from build123d import *

# Parameters (mm, degrees)
SKETCH1_W           = 155
SKETCH1_H           = 55
SKETCH1_R           = 3.25
BOSS_EXTRUDE1_DEPTH = 10
CUT_EXTRUDE1_DEPTH  = 7
SKETCH3_R           = 2.5
CUT_EXTRUDE2_DEPTH  = 10
FILLET1_R           = 3


with BuildPart() as part:
    # Sketch1 → Boss-Extrude1 (new body)
    with BuildSketch(Plane.XY):
        with Locations((2.15707133, 4.04038984)):
            Rectangle(SKETCH1_W, SKETCH1_H)
        with Locations((-45.34292867, 4.04038984)):
            Circle(SKETCH1_R, mode=Mode.SUBTRACT)
        with Locations((-8.34292867, 4.04038984)):
            Circle(SKETCH1_R, mode=Mode.SUBTRACT)
        with Locations((55.65707133, 6.54038984)):
            Circle(SKETCH1_R, mode=Mode.SUBTRACT)
    extrude(amount=BOSS_EXTRUDE1_DEPTH)

    # Sketch2 → Cut-Extrude1 (cut)
    with BuildSketch(Plane.XY.offset(10)):
        with BuildLine():
            Line((-75.34292867, 31.54038984), (-63.34292867, 31.54038984))
            Line((-63.34292867, 31.54038984), (-63.34292867, 24.04038984))
            ThreePointArc((-63.34292867, 24.04038984), (-64.660948155, 20.858409325), (-67.84292867, 19.54038984))
            Line((-67.84292867, 19.54038984), (-75.34292867, 19.54038984))
            Line((-75.34292867, 19.54038984), (-75.34292867, 31.54038984))
        make_face()
        with BuildLine():
            Line((-75.34292867, -23.45961016), (-63.34292867, -23.45961016))
            Line((-63.34292867, -23.45961016), (-63.34292867, -15.95961016))
            ThreePointArc((-63.34292867, -15.95961016), (-64.660948155, -12.777629645), (-67.84292867, -11.45961016))
            Line((-67.84292867, -11.45961016), (-75.34292867, -11.45961016))
            Line((-75.34292867, -11.45961016), (-75.34292867, -23.45961016))
        make_face()
        with BuildLine():
            Line((79.65707133, -23.45961016), (67.65707133, -23.45961016))
            Line((67.65707133, -23.45961016), (67.65707133, -15.95961016))
            ThreePointArc((67.65707133, -15.95961016), (68.975090815, -12.777629645), (72.15707133, -11.45961016))
            Line((72.15707133, -11.45961016), (79.65707133, -11.45961016))
            Line((79.65707133, -11.45961016), (79.65707133, -23.45961016))
        make_face()
        with BuildLine():
            Line((79.65707133, 31.54038984), (67.65707133, 31.54038984))
            Line((67.65707133, 31.54038984), (67.65707133, 24.04038984))
            ThreePointArc((67.65707133, 24.04038984), (68.975090815, 20.858409325), (72.15707133, 19.54038984))
            Line((72.15707133, 19.54038984), (79.65707133, 19.54038984))
            Line((79.65707133, 19.54038984), (79.65707133, 31.54038984))
        make_face()
    extrude(amount=-CUT_EXTRUDE1_DEPTH, mode=Mode.SUBTRACT)

    # Sketch3 → Cut-Extrude2 (cut)
    with BuildSketch(Plane.XY.offset(3)):
        with Locations((-68.34292867, -16.45961016)):
            Circle(SKETCH3_R)
        with Locations((72.65707133, -16.45961016)):
            Circle(SKETCH3_R)
        with Locations((72.65707133, 24.54038984)):
            Circle(SKETCH3_R)
        with Locations((-68.34292867, 24.54038984)):
            Circle(SKETCH3_R)
    extrude(amount=-CUT_EXTRUDE2_DEPTH, mode=Mode.SUBTRACT)

    # Fillet1
    fillet1_edges = [part.edges().sort_by_distance(p)[0] for p in [
        (79.65707133, 19.54038984, 6.5),
        (67.65707133, 31.54038984, 6.5),
        (79.65707133, -11.45961016, 6.5),
        (67.65707133, -23.45961016, 6.5),
        (-75.34292867, -11.45961016, 6.5),
        (-63.34292867, -23.45961016, 6.5),
        (-75.34292867, 19.54038984, 6.5),
        (-63.34292867, 31.54038984, 6.5),
    ]]
    fillet(fillet1_edges, radius=FILLET1_R)


solid = part.part
Can you work these out from the model? Positions are in its coordinate system, mm. A direction names the side the tool comes from. Give positions to 0.01 mm unless a question says otherwise; leave off trailing zeros. Order: outer loops, then holes, each group sorted by start corner. A loop starts at its lowest first (then second) coordinate and runs counter-clockwise, first axis right, second up. Notation, with made-up numbers: M 87.5,55.25 L 116.5,55.25 A23 ccw 116.5,85.25 Z; hole C -19,17.25 d6. An arc over 180 degrees is marked long. Use a Markdown table: item, result. Add a question column.
Item 1: If I drill on L1, parallel to X at y = 1.5, z = 5.25; L2, parallel to X at y = 6.5, z = 1.75; L3, parallel to X at y = 7.5, z = 8.75, over which ranges is the centre line in solid material (lowest first)? Write a range as [from, to].
Item 2: Suppose I cut it at A-A (z = 5.75). List the corners of the cut face in (x, y) for me, then the cut area to 3 significant figures.
Item 3: Will these pins go through, and if not, where does the flat tip stop? pin 1 (5 mm diameter, centred on x = -70, z = 7, fed in from -Y); pin 2 (5 mm diameter, centred on x = -70.5, z = 6, fed in from +Y); pin 3 (2 mm diameter, centred on y = -19, z = 6.5, fed in from +X); pin 4 (3 mm diameter, centred on x = -68.34, y = 24.54, fed in from -Z).
Item 4: We'd pull the mould along Y, two halves only. Please class faces 4 (the flat face through (74, 19.54, 7)), 5 (the flat face through (74, 27, 3)), 6 (the flat face through (1, -23.46, 5)), 7 (the cylindrical face through (70.16, -16.35, 1.52)): +Y half, -Y half, draft (parallel to the pull), parting line (faces both ways), or undercut.
Item 5: For faces 1 (the flat face through (67.657, -18, 7)), 2 (the flat face through (-63.343, -18, 7)), 3 (the cylindrical face through (58.66, 5.3, 4.93)), which set-ups out of +Z, -Z, +X, -X, +Y, -Y let a thin tool reach every point of the face, with its end or its side?
Answer sheet:
| question | item | result |
|---|---|---|
| 1 | L1 | x = [-75.34, -47.37], [-43.32, -10.37], [-6.32, 79.66] |
| 1 | L2 | x = [-75.34, -47.47], [-43.22, -10.47], [-6.22, 52.41], [58.91, 79.66] |
| 1 | L3 | x = [-75.34, 52.55], [58.76, 79.66] |
| 2 | outline | M -75.34,-8.46 A3 ccw -72.34,-11.46 L -67.84,-11.46 A4.5 cw -63.34,-15.96 L -63.34,-20.46 A3 ccw -60.34,-23.46 L 64.66,-23.46 A3 ccw 67.66,-20.46 L 67.66,-15.96 A4.5 cw 72.16,-11.46 L 76.66,-11.46 A3 ccw 79.66,-8.46 L 79.66,16.54 A3 ccw 76.66,19.54 L 72.16,19.54 A4.5 cw 67.66,24.04 L 67.66,28.54 A3 ccw 64.66,31.54 L -60.34,31.54 A3 ccw -63.34,28.54 L -63.34,24.04 A4.5 cw -67.84,19.54 L -72.34,19.54 A3 ccw -75.34,16.54 Z; hole C -45.34,4.04 d6.5; hole C -8.34,4.04 d6.5; hole C 55.66,6.54 d6.5 |
| 2 | area | 7,850 mm² |
| 3 | pin 1 | stops at y = -11.47 |
| 3 | pin 2 | stops at y = 19.54 |
| 3 | pin 3 | stops at x = 67.66 |
| 3 | pin 4 | passes through |
| 4 | face 4 | +Y half |
| 4 | face 5 | draft |
| 4 | face 6 | -Y half |
| 4 | face 7 | undercut |
| 5 | face 1 | +Z, +X, -Y |
| 5 | face 2 | +Z, -X, -Y |
| 5 | face 3 | +Z, -Z |
